```python
from build123d import *

# Parameters (mm, degrees)
SKETCH1_W                  = 184.15
SKETCH1_H                  = 63.5
BOSS_EXTRUDE1_DEPTH        = 6.35
SKETCH3_R                  = 14.605
CUT_EXTRUDE1_DEPTH         = 98.602206046
F_10_CLEARANCE_HOLE1_D     = 5.1054
F_6_5_6_5_DIAMETER_HOLE3_D = 6.5
SKETCH29_R                 = 15.875
CUT_EXTRUDE5_DEPTH         = 3.175
F_10_CLEARANCE_HOLE2_D     = 5.1054
SKETCH36_R                 = 2.54
CUT_EXTRUDE6_DEPTH         = 98.602206046
SKETCH37_W                 = 25.4
SKETCH37_H                 = 25.4
CUT_EXTRUDE7_DEPTH         = 98.602206046
SKETCH38_W                 = 25.4
SKETCH38_H                 = 25.4
CUT_EXTRUDE8_DEPTH         = 98.602206046


with BuildPart() as part:
    # Sketch1 → Boss-Extrude1 (new body)
    with BuildSketch(Plane(origin=(0, 0, 0), x_dir=(1, 0, 0), z_dir=(0, 1, 0))):
        Rectangle(SKETCH1_W, SKETCH1_H)
    extrude(amount=BOSS_EXTRUDE1_DEPTH)

    # Sketch3 → Cut-Extrude1 (cut, through all)
    with BuildSketch(Plane(origin=(0, 6.35, 0), x_dir=(1, 0, 0), z_dir=(0, 1, 0))):
        with Locations(Location((0, 0, 0), (0, 0, 270))):
            Circle(SKETCH3_R)
    extrude(amount=-CUT_EXTRUDE1_DEPTH, mode=Mode.SUBTRACT)

    # #10 Clearance Hole1 (through all)
    with Locations(Plane(origin=(0, 0, 0), x_dir=(-1, 0, 0), z_dir=(0, -1, 0))):
        with Locations((0, -25.4), (0, 25.4)):
            Hole(F_10_CLEARANCE_HOLE1_D / 2)

    # Ø6.5 (6.5) Diameter Hole3 (through all)
    with Locations(Plane(origin=(0, 0, 0), x_dir=(-1, 0, 0), z_dir=(0, -1, 0))):
        with Locations((58.039, 0), (-58.039, 0)):
            Hole(F_6_5_6_5_DIAMETER_HOLE3_D / 2)

    # Sketch29 → Cut-Extrude5 (cut)
    with BuildSketch(Plane(origin=(0, 6.35, 0), x_dir=(1, 0, 0), z_dir=(0, 1, 0))):
        with Locations(Location((0, 0, 0), (0, 0, 270))):
            Circle(SKETCH29_R)
    extrude(amount=-CUT_EXTRUDE5_DEPTH, mode=Mode.SUBTRACT)

    # #10 Clearance Hole2 (through all)
    with Locations(Plane(origin=(0, 6.35, 0), x_dir=(1, 0, 0), z_dir=(0, 1, 0))):
        with Locations((-82.55, 19.05), (-82.55, -19.05), (82.55, -19.05), (82.55, 19.05), (-82.55, 0), (82.55, 0)):
            Hole(F_10_CLEARANCE_HOLE2_D / 2)

    # Sketch36 → Cut-Extrude6 (cut, through all)
    with BuildSketch(Plane.XZ):
        with Locations(Location((-21.329210467, 13.7922, 0), (0, 0, 270))):
            Circle(SKETCH36_R)
        with Locations(Location((21.329210467, -13.7922, 0), (0, 0, 270))):
            Circle(SKETCH36_R)
    extrude(amount=-CUT_EXTRUDE6_DEPTH, mode=Mode.SUBTRACT)

    # Sketch37 → Cut-Extrude7 (cut, through all)
    with BuildSketch(Plane(origin=(0, 6.35, 0), x_dir=(1, 0, 0), z_dir=(0, 1, 0))):
        with Locations((-58.039, 0)):
            Rectangle(SKETCH37_W, SKETCH37_H)
    extrude(amount=-CUT_EXTRUDE7_DEPTH, mode=Mode.SUBTRACT)

    # Sketch38 → Cut-Extrude8 (cut, through all)
    with BuildSketch(Plane(origin=(0, 6.35, 0), x_dir=(1, 0, 0), z_dir=(0, 1, 0))):
        with Locations((58.039, 0)):
            Rectangle(SKETCH38_W, SKETCH38_H)
    extrude(amount=-CUT_EXTRUDE8_DEPTH, mode=Mode.SUBTRACT)


solid = part.part
```
The model under review builds one solid part; all positions refer to its coordinate system, in mm. A direction names the side the tool comes from. Coordinates: 2 decimals unless noted, no trailing zeros. Write each loop counter-clockwise with the first axis right and the second up, starting at its lowest first coordinate (ties: lowest second). Pieces come first, ordered by that corner, then holes. Notation, with made-up numbers: (41, -23) - (61, -23) arc R11 cw to (61, -13) - close; hole circle Ø5 at (1.5, 47.25). An arc over 180 degrees is marked (long way). Answer in a Markdown table with one row per item. Add a question column.
Q1. Draft analysis for pull direction Z (two halves, no side actions). For faces 4 (the face through (1.372, 3.219, -27.552)), 5 (the face through (-1, 3, -31.75)), 6 (the face through (19, 6.35, 0)), state which applies: +Z half, -Z half, draft (parallel to the pull), parting line (faces both ways), or undercut.
Q2. Consider section A-A on z = 0. Give the boundary of the cut face in (x, y) (3 decimals).
Q3. Consider section B-B on x = 0. Give the boundary of the cut face in (y, z) (3 decimals), then the cut area to 3 significant figures.
Q4. Consider section C-C on z = -19.05. Give the boundary of the cut face in (x, y) (3 decimals), then the cut area to 3 significant figures.
Q5. Consider section D-D on y = 4.75. Give the number of separate pieces and of enclosed holes in the cut face, then the cut area to 3 significant figures.
Q6. For faces 1 (the face through (-1, 0, -15)), 2 (the face through (-58, 3, -12.7)), 3 (the face through (-13, 3.175, 7)), list the 3-axis set-ups (+Z, -Z, +X, -X, +Y, -Y) from which the entire face can be reached by the end or side of a thin tool; tool diameter is ignored.
Q7. To check wall thickness, follow line 1 along Z through (x, y) = (-82.55, 2); line 2 along X through (y, z) = (4.25, -19.05) (3 decimals); line 3 along Z through (x, y) = (-64.5, 4.75). State the ranges of each line that lie inside material, in increasing order. Write a range as from..to.
Answers below:
| question | item | result |
|---|---|---|
| 1 | face 4 | undercut |
| 1 | face 5 | -Z half |
| 1 | face 6 | draft |
| 2 | outline | (-92.075, 0) - (-85.103, 0) - (-85.103, 6.35) - (-92.075, 6.35) - close; (-79.997, 0) - (-70.739, 0) - (-70.739, 6.35) - (-79.997, 6.35) - close; (-45.339, 0) - (-14.605, 0) - (-14.605, 3.175) - (-15.875, 3.175) - (-15.875, 6.35) - (-45.339, 6.35) - close; (14.605, 0) - (45.339, 0) - (45.339, 6.35) - (15.875, 6.35) - (15.875, 3.175) - (14.605, 3.175) - close; (70.739, 0) - (79.997, 0) - (79.997, 6.35) - (70.739, 6.35) - close; (85.103, 0) - (92.075, 0) - (92.075, 6.35) - (85.103, 6.35) - close |
| 3 | outline | (0, -31.75) - (6.35, -31.75) - (6.35, -27.953) - (0, -27.953) - close; (0, -22.847) - (6.35, -22.847) - (6.35, -15.875) - (3.175, -15.875) - (3.175, -14.605) - (0, -14.605) - close; (0, 14.605) - (3.175, 14.605) - (3.175, 15.875) - (6.35, 15.875) - (6.35, 22.847) - (0, 22.847) - close; (0, 27.953) - (6.35, 27.953) - (6.35, 31.75) - (0, 31.75) - close |
| 3 | area | 145 mm² |
| 4 | outline | (-92.075, 0) - (-85.103, 0) - (-85.103, 6.35) - (-92.075, 6.35) - close; (-79.997, 0) - (79.997, 0) - (79.997, 6.35) - (-79.997, 6.35) - close; (85.103, 0) - (92.075, 0) - (92.075, 6.35) - (85.103, 6.35) - close |
| 4 | area | 1,100 mm² |
| 5 | separate pieces | 1 |
| 5 | enclosed holes | 13 |
| 5 | area | 9,410 mm² |
| 6 | face 1 | +Z, -Z, +X, -X, -Y |
| 6 | face 2 | +Y, -Y |
| 6 | face 3 | +Y |
| 7 | line 1 | -31.75..-21.6, -16.5..-2.55, 2.55..16.5, 21.6..31.75 |
| 7 | line 2 | -92.075..-85.103, -79.997..79.997, 85.103..92.075 |
| 7 | line 3 | -31.75..-12.7, 12.7..31.75 |
